Verification items for this drawing (mm, ordinates from the low corner). Coordinates: 2 decimals unless noted, no trailing zeros. Write each loop counter-clockwise with the first axis right and the second up, starting at its lowest first coordinate (ties: lowest second). Pieces come first, ordered by that corner, then holes. Notation, with made-up numbers: (38, -39) -> (60, -39) arc R26 ccw to (60, -2) -> close; hole circle Ø5 at (29, -4). An arc over 180 degrees is marked (long way). Use CSV: the item, a comma, the result in double quotes.
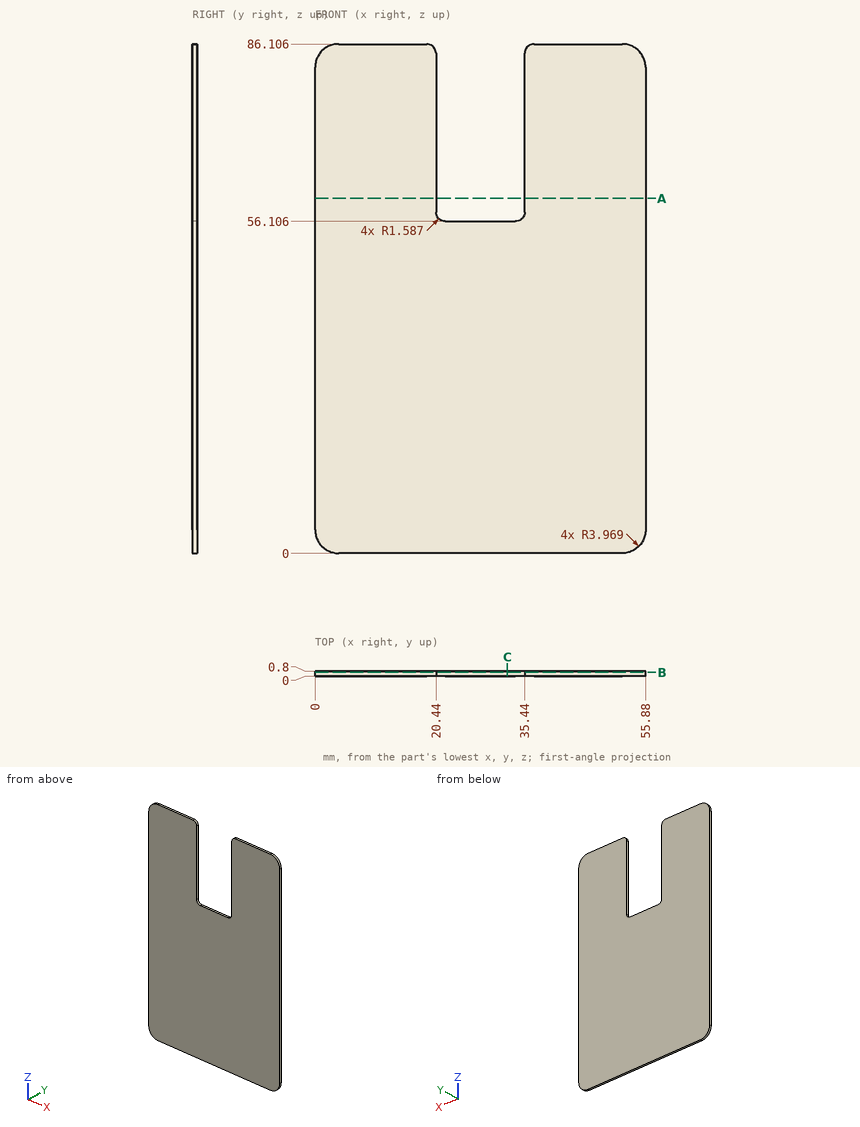
1) Cross-section at A-A (z = 60). Record the boundary of the cut face in (x, y).
Return value:
outline,"(0, 0) -> (20.44, 0) -> (20.44, 0.8) -> (0, 0.8) -> close; (35.44, 0) -> (55.88, 0) -> (55.88, 0.8) -> (35.44, 0.8) -> close"
2) Cross-section at B-B (y = 0.6). Record the boundary of the cut face in (x, z) (1 decimal), plus the area to 3 significant figures.
Return value:
outline,"(0, 4) arc R4 ccw to (4, 0) -> (51.9, 0) arc R4 ccw to (55.9, 4) -> (55.9, 82.1) arc R4 ccw to (51.9, 86.1) -> (37, 86.1) arc R1.6 ccw to (35.4, 84.5) -> (35.4, 57.7) arc R1.6 cw to (33.9, 56.1) -> (22, 56.1) arc R1.6 cw to (20.4, 57.7) -> (20.4, 84.5) arc R1.6 ccw to (18.9, 86.1) -> (4, 86.1) arc R4 ccw to (0, 82.1) -> close"
area,"4,350 mm2"
3) Cross-section at C-C (x = 32.5). Record the boundary of the cut face in (y, z) (1 decimal).
Return value:
outline,"(0, 0) -> (0.8, 0) -> (0.8, 56.1) -> (0, 56.1) -> close"
4) Scan lines: L1, parallel to X at y = 0.7, z = 65; L2, parallel to X at y = 0.65, z = 83 (1 decimal); L3, parallel to Z at x = 33, y = 0.7 (1 decimal). Record each from-to range of solid material in increasing order.
Return value:
L1,"0 to 20.44, 35.44 to 55.88"
L2,"0.1 to 20.4, 35.4 to 55.8"
L3,"0 to 56.1"
5) Gauge pin test, flat end, axial feed: pin 1 (10 mm diameter, centred on x = 17.5, z = 74, fed in from -Y). Record the tip position at first contact, or that the pin passes through.
Return value:
pin 1,"y = 0"
